Geometry: final body of the model. Coordinates: model frame, mm. Round coordinates to 2 decimals unless told otherwise and drop trailing zeros. Write each loop counter-clockwise with the first axis right and the second up, starting at its lowest first coordinate (ties: lowest second). Pieces come first, ordered by that corner, then holes. Notation, with made-up numbers: (-20, -15.75) - (-1, -15.75) arc R22 cw to (-1, 15.25) - close; hole circle Ø11 at (-16.5, 28.5). An arc over 180 degrees is marked (long way). Use a Markdown table: item, result. Add a question column.
```python
from build123d import *

# Parameters (mm, degrees)
SKETCH1_R           = 6.5
SKETCH1_R_2         = 2.75
BOSS_EXTRUDE1_DEPTH = 5


with BuildPart() as part:
    # Sketch1 → Boss-Extrude1 (new body)
    with BuildSketch(Plane.XY):
        with BuildLine():
            Line((-23.503678525, 19.646734505), (-23.503678525, 12.353265495))
            Line((-23.503678525, 12.353265495), (-4.861111111, 4.4839417))
            ThreePointArc((-4.861111111, 4.4839417), (0, 3.5), (4.861111111, 4.4839417))
            Line((4.861111111, 4.4839417), (23.503678525, 12.353265495))
            Line((23.503678525, 12.353265495), (23.503678525, 19.646734505))
            Line((23.503678525, 19.646734505), (4.861111111, 27.5160583))
            ThreePointArc((4.861111111, 27.5160583), (0, 28.5), (-4.861111111, 27.5160583))
            Line((-4.861111111, 27.5160583), (-23.503678525, 19.646734505))
        make_face()
        with Locations((0, 16)):
            Circle(SKETCH1_R, mode=Mode.SUBTRACT)
        with Locations((-18, 16)):
            Circle(SKETCH1_R_2, mode=Mode.SUBTRACT)
        with Locations((18, 16)):
            Circle(SKETCH1_R_2, mode=Mode.SUBTRACT)
    extrude(amount=BOSS_EXTRUDE1_DEPTH)


solid = part.part
```
1) Material intervals for L1, parallel to X at y = 16.25, z = 1.3; L2, parallel to X at y = 14.5, z = 1; L3, parallel to Y at x = 0, z = 1.9, sorted ascending. Write a range as from..to.
2) Section C-C, the plane z = 4.15. Return the cut outline in (x, y).
3) Pin query (flat end, axial travel): P1, Ø2, axis at x = 11, z = 2.5, coming from the -Y side; P2, Ø1, axis at y = 25.5, z = 3, coming from the +X side; P3, Ø2, axis at y = 22.5, z = 3, coming from the +X side. Return the tip coordinate at first contact, or that it passes through.
4) Section D-D, the plane x = 18. Return the cut outline in (y, z), then the cut area to 3 significant figures.
5) Section B-B, the plane y = 16. Return the cut outline in (x, z).
6) Draft query along X for faces 1 (the cylindrical face through (17.642, 18.727, 2.465)), 2 (the flat face through (14.052, 8.364, 2.465)), 3 (the flat face through (-6, 11, 5)). Return one class per face: released by +X, released by -X, zero draft, split by the parting line, or undercut.
7) Section A-A, the plane x = 0. Return the cut outline in (y, z).
Output values:
| question | item | result |
|---|---|---|
| 1 | L1 | x = -23.5..-20.74, -15.26..-6.5, 6.5..15.26, 20.74..23.5 |
| 1 | L2 | x = -23.5..-20.3, -15.7..-6.32, 6.32..15.7, 20.3..23.5 |
| 1 | L3 | y = 3.5..9.5, 22.5..28.5 |
| 2 | outline | (-23.5, 12.35) - (-4.86, 4.48) arc R12.5 ccw to (4.86, 4.48) - (23.5, 12.35) - (23.5, 19.65) - (4.86, 27.52) arc R12.5 ccw to (-4.86, 27.52) - (-23.5, 19.65) - close; hole circle Ø5.5 at (-18, 16); hole circle Ø13 at (0, 16); hole circle Ø5.5 at (18, 16) |
| 3 | P1 | stops at y = 6.65 |
| 3 | P2 | stops at x = 10.82 |
| 3 | P3 | stops at x = 19.11 |
| 4 | outline | (10.03, 0) - (13.25, 0) - (13.25, 5) - (10.03, 5) - close; (18.75, 0) - (21.97, 0) - (21.97, 5) - (18.75, 5) - close |
| 4 | area | 32.2 mm^2 |
| 5 | outline | (-23.5, 0) - (-20.75, 0) - (-20.75, 5) - (-23.5, 5) - close; (-15.25, 0) - (-6.5, 0) - (-6.5, 5) - (-15.25, 5) - close; (6.5, 0) - (15.25, 0) - (15.25, 5) - (6.5, 5) - close; (20.75, 0) - (23.5, 0) - (23.5, 5) - (20.75, 5) - close |
| 6 | face 1 | undercut |
| 6 | face 2 | released by +X |
| 6 | face 3 | zero draft |
| 7 | outline | (3.5, 0) - (9.5, 0) - (9.5, 5) - (3.5, 5) - close; (22.5, 0) - (28.5, 0) - (28.5, 5) - (22.5, 5) - close |
